Could you check a few things on this model? Use its own coordinates, in mm. A direction names the side the tool comes from. Give positions to 0.01 mm unless a question says otherwise; leave off trailing zeros. Order: outer loops, then holes, each group sorted by start corner. A loop starts at its lowest first (then second) coordinate and runs counter-clockwise, first axis right, second up. Notation, with made-up numbers: (10, 70.25) -> (63, 70.25) arc R28 cw to (63, 90.25) -> close; hole circle Ø3 at (12, 79). An arc over 180 degrees is marked (long way). Answer as CSV lines item,"result". Start each with the question number.
(1) I want a section at A-A (z = 0). Please give me the cut outline in (x, y).
(2) I want a section at D-D (x = 0). Please give me the cut outline in (y, z), plus the area to 3 significant figures.
(3) On a 3-axis mill with a long thin cutter (end or side, diameter ignored), from which of +Z, -Z, +X, -X, +Y, -Y can I reach the whole of each face in a straight line? I mean faces 1 (the face through (-0.75, 10, -3)), 2 (the face through (-5, 21, -1)), 3 (the face through (-6.5, 14, -5)), 4 (the face through (5.23, 8.02, -9.39)). Say none if no direction works.
(4) I want a section at B-B (z = -5). Please give me the cut outline in (x, y).
(5) I need wall thicknesses on L1, parallel to Y at x = 3.45, z = -5; L2, parallel to Y at x = -9.25, z = -2; L3, parallel to Z at x = -5.75, y = 25. Which ranges of each line are inside material? Lowest first, please.
(6) I want a section at C-C (y = 11.25). Please give me the cut outline in (x, z).
(7) Will these pins go through, and if not, where does the flat tip stop? pin 1 Ø6 at (x, y) = (-8, 5) entering from -Z; pin 2 Ø3 at (x, z) = (-6, -3.5) entering from +Y; pin 3 Ø3.5 at (x, y) = (-9, 17) entering from -Z.
(8) We'd pull the mould along Z, two halves only. Please class faces 5 (the face through (-2.65, 10.35, -0.05)), 6 (the face through (8, 7.5, -4)), 7 (the face through (-1.07, 10.65, -8.14)): released by +Z, released by -Z, zero draft, split by the parting line, or undercut.
```python
from build123d import *

# Parameters (mm, degrees)
SKICA1_R                      = 10.75
SKICA1_R_2                    = 2.65
P_IDAT_VYSUNUT_M1_DEPTH       = 21
ODEBRAT_VYSUNUT_M1_DEPTH      = 26.925373671
ODEBRAT_VYSUNUT_M1_DEPTH_BACK = 26.925373671
SKICA2_W                      = 1.5
SKICA2_H                      = 14.75
ODEBRAT_START                 = -13.5
ODEBRAT_VYSUNUT_M2_DEPTH      = 13.5
SKICA5_R                      = 1.75
ODEBRAT_VYSUNUT_M3_DEPTH      = 30.22541702
P_IDAT_VYSUNUT_M3_DEPTH       = 10
SKICA2_2_W                    = 1.5
SKICA2_2_H                    = 14.75
ODEBRAT_VYSUNUT_M4_DEPTH      = 28.95643933
P_IDAT_VYSUNUT_M6_DEPTH       = 20
ZKOSEN_1_SIZE                 = 1
SKICA9_W                      = 20
SKICA9_H                      = 2.57342531
SKICA9_H_2                    = 5
P_IDAT_VYSUNUT_M5_DEPTH       = 1
SKICA11_W                     = 1.5
SKICA11_H                     = 1
ODEBRAT_VYSUNUT_M5_DEPTH      = 30.41747401
ODEBRAT_VYSUNUT_M6_DEPTH      = 30.41747401
P_IDAT_VYSUNUT_M7_DEPTH       = 20
SKICA15_W                     = 1
SKICA15_H                     = 1
ODEBRAT_VYSUNUT_M8_DEPTH      = 43.326853179


with BuildPart() as part:
    # Skica1 → Přidat vysunutím1 (new body)
    with BuildSketch(Plane(origin=(0, 0, 0), x_dir=(1, 0, 0), z_dir=(0, 1, 0))):
        with Locations(Location((0, 0, 0), (0, 0, 90))):
            Circle(SKICA1_R)
        with Locations(Location((0, 0, 0), (0, 0, 90))):
            Circle(SKICA1_R_2, mode=Mode.SUBTRACT)
    extrude(amount=P_IDAT_VYSUNUT_M1_DEPTH)

    # Skica2 → Odebrat vysunutím1 (cut, two sides: drawn at the far end of the back side and taken through both)
    with BuildSketch(Plane(origin=(0, 21, 0), x_dir=(1, 0, 0), z_dir=(0, 1, 0)).offset(-ODEBRAT_VYSUNUT_M1_DEPTH_BACK)):
        with Locations((0, 3.375)):
            Rectangle(SKICA2_W, SKICA2_H)
    extrude(amount=ODEBRAT_VYSUNUT_M1_DEPTH + ODEBRAT_VYSUNUT_M1_DEPTH_BACK, mode=Mode.SUBTRACT)

    # Skica4 → Odebrat vysunutím2 (cut)
    with BuildSketch(Plane(origin=(0, 21, 0), x_dir=(1, 0, 0), z_dir=(0, 1, 0)).offset(ODEBRAT_START)):
        with BuildLine():
            ThreePointArc((-6.5, 8.562271895), (-9.334363095, 5.332182069), (-10.677078252, 1.25))
            Line((-10.677078252, 1.25), (-6.5, 1.25))
            Line((-6.5, 1.25), (-6.5, 8.562271895))
        make_face()
        with BuildLine():
            Line((6.5, 1.25), (10.677078252, 1.25))
            ThreePointArc((10.677078252, 1.25), (9.334363095, 5.332182069), (6.5, 8.562271895))
            Line((6.5, 8.562271895), (6.5, 1.25))
        make_face()
    extrude(amount=ODEBRAT_VYSUNUT_M2_DEPTH, mode=Mode.SUBTRACT)

    # Skica5 → Odebrat vysunutím3 (cut, through all)
    with BuildSketch(Plane.ZY.offset(6.5)):
        with Locations((-5, 11.25)):
            Circle(SKICA5_R)
    extrude(amount=-ODEBRAT_VYSUNUT_M3_DEPTH, mode=Mode.SUBTRACT)

    # Skica6 → Přidat vysunutím3 (add, symmetric)
    with BuildSketch(Plane(origin=(0, 0, 0), x_dir=(0, 0, -1), z_dir=(1, 0, 0))):
        Polygon((-15, 31), (-10, 31), (-10, 21), (-3.94493346, 21), (-3.94493346, 7.5), (-15, 16.776302257), align=None)
    extrude(amount=P_IDAT_VYSUNUT_M3_DEPTH, both=True)

    # Skica2<2> → Odebrat vysunutím4 (cut, through all)
    with BuildSketch(Plane(origin=(0, 21, 0), x_dir=(1, 0, 0), z_dir=(0, 1, 0))):
        with Locations((0, 3.375)):
            Rectangle(SKICA2_2_W, SKICA2_2_H)
    extrude(amount=-ODEBRAT_VYSUNUT_M4_DEPTH, mode=Mode.SUBTRACT)

    # Skica8 → Přidat vysunutím6 (add)
    with BuildSketch(Plane(origin=(10, 0, 0), x_dir=(0, 0, -1), z_dir=(1, 0, 0))):
        Polygon((-15, 16.776302257), (-17.57342531, 18.935662485), (-17.57342531, 21), (-15, 21), align=None)
    extrude(amount=-P_IDAT_VYSUNUT_M6_DEPTH)

    # Zkosení1
    zkosen_1_edges = [part.edges().sort_by_distance(p)[0] for p in [
        (10, 31, 12.5),
        (-10, 31, 12.5),
    ]]
    chamfer(zkosen_1_edges, length=ZKOSEN_1_SIZE)

    # Skica9 → Přidat vysunutím5 (add)
    with BuildSketch(Plane(origin=(0, 21, 0), x_dir=(1, 0, 0), z_dir=(0, 1, 0))):
        with Locations((0, -16.286712655)):
            Rectangle(SKICA9_W, SKICA9_H)
        with Locations((0, -7.5)):
            Rectangle(SKICA9_W, SKICA9_H_2)
    extrude(amount=P_IDAT_VYSUNUT_M5_DEPTH)

    # Skica11 → Odebrat vysunutím5 (cut, through all)
    with BuildSketch(Plane(origin=(0, 21, 0), x_dir=(1, 0, 0), z_dir=(0, 1, 0))):
        with Locations((0, -4.5)):
            Rectangle(SKICA11_W, SKICA11_H)
    extrude(amount=-ODEBRAT_VYSUNUT_M5_DEPTH, mode=Mode.SUBTRACT)

    # Skica12 → Odebrat vysunutím6 (cut, through all)
    with BuildSketch(Plane(origin=(0, 21, 0), x_dir=(1, 0, 0), z_dir=(0, 1, 0))):
        Polygon((0, 0), (-1.415264349, 10.75), (1.415264349, 10.75), align=None)
    extrude(amount=-ODEBRAT_VYSUNUT_M6_DEPTH, mode=Mode.SUBTRACT)

    # Skica13 → Přidat vysunutím7 (add)
    with BuildSketch(Plane(origin=(10, 0, 0), x_dir=(0, 0, -1), z_dir=(1, 0, 0))):
        Polygon((-17.57342531, 18.935662485), (-20, 20.971800413), (-20, 22), (-17.57342531, 22), align=None)
    extrude(amount=-P_IDAT_VYSUNUT_M7_DEPTH)

    # Skica15 → Odebrat vysunutím8 (cut, through all)
    with BuildSketch(Plane.ZY.offset(10)):
        with Locations((9.5, 21.5)):
            Rectangle(SKICA15_W, SKICA15_H)
        with Locations((15.5, 21.5)):
            Rectangle(SKICA15_W, SKICA15_H)
    extrude(amount=-ODEBRAT_VYSUNUT_M8_DEPTH, mode=Mode.SUBTRACT)


solid = part.part
```
Final values:
1,outline,"(-10.75, 0) -> (-2.65, 0) -> (-2.65, 21) -> (-10.75, 21) -> close; (2.65, 0) -> (10.75, 0) -> (10.75, 21) -> (2.65, 21) -> close"
2,outline,"(0, 5) -> (22, 5) -> (22, 9) -> (21, 9) -> (21, 10) -> (31, 10) -> (31, 15) -> (21, 15) -> (21, 16) -> (22, 16) -> (22, 20) -> (20.97, 20) -> (13.21, 10.75) -> (0, 10.75) -> close"
2,area,"215 mm²"
3,face 1,"-Z, +Y, -Y"
3,face 2,"-Z, +X, -X, +Y"
3,face 3,"-Z, -X, +Y"
3,face 4,"-Y"
4,outline,"(-9.52, 0) -> (-0.75, 0) -> (-0.75, 9.5) -> (-6.5, 9.5) -> (-6.5, 7.5) -> (-9.52, 7.5) -> close; (-6.5, 13) -> (-0.75, 13) -> (-0.75, 21) -> (-6.5, 21) -> close; (0.75, 0) -> (9.52, 0) -> (9.52, 7.5) -> (6.5, 7.5) -> (6.5, 9.5) -> (0.75, 9.5) -> close; (0.75, 13) -> (6.5, 13) -> (6.5, 21) -> (0.75, 21) -> close"
5,L1,"0 to 9.5, 13 to 21"
5,L2,"0 to 7.5"
5,L3,"10 to 15"
6,outline,"(-10.68, -1.25) -> (-6.5, -1.25) -> (-6.5, -3.25) -> (-0.75, -3.25) -> (-0.75, -2.54) arc R2.65 cw to (-0.75, 2.54) -> (-0.75, 5) -> (0.75, 5) -> (0.75, 2.54) arc R2.65 cw to (0.75, -2.54) -> (0.75, -3.25) -> (6.5, -3.25) -> (6.5, -1.25) -> (10.68, -1.25) arc R10.75 ccw to (10, 3.94) -> (10, 8.41) -> (6.69, 8.41) arc R10.75 ccw to (-6.69, 8.41) -> (-10, 8.41) -> (-10, 3.94) arc R10.75 ccw to start; (-6.5, -8.56) arc R10.75 ccw to (-1.4, -10.66) -> (-0.89, -6.75) -> (-6.5, -6.75) -> close; (0.89, -6.75) -> (1.4, -10.66) arc R10.75 ccw to (6.5, -8.56) -> (6.5, -6.75) -> close"
7,pin 1,"z = -9.52"
7,pin 2,"y = 21"
7,pin 3,"z = -1.25"
8,face 5,"undercut"
8,face 6,"zero draft"
8,face 7,"released by -Z"
